Autodesk Inventor part; units mm, degrees
ref_plane "YZ Plane" through (0, 0, 0) normal (1, 0, 0) x (0, 1, 0)
ref_plane "XZ Plane" through (0, 0, 0) normal (0, 1, 0) x (-1, 0, 0)
ref_plane "XY Plane" through (0, 0, 0) normal (0, 0, 1) x (1, 0, 0)
sketch "Sketch1" plane through (0, 0, 0) normal (0, 1, 0) x (-1, 0, 0)
  line L0 (0, 0) -> (0, -42)
  line L1 (0, -42) -> (12, -42)
  line L2 (12, -42) -> (12, 0)
  line L3 (12, 0) -> (0, 0)
  line L4 (0, -21) -> (0, -26)
  line L5 (0, -21) -> (0, -16)
  line L6 (0, -16) -> (0, -19)
  line L7 (0, -16) -> (0, -13)
  line L8 (0, -26) -> (0, -23)
  line L9 (0, -26) -> (0, -29)
  line L10 (0, -29) -> (12, -29)
  line L11 (0, -13) -> (12, -13)
  line L12 (6.4, -16) -> (12, -16)
  line L13 (6.4, -26) -> (12, -26)
  line L14 (12, -16) -> (8, -16)
  circle A0 centre (8, -16) radius 1.6
  circle A1 centre (8, -26) radius 1.6
  line L15 (12, -26) -> (8, -26)
  dimension "d9" = 3.2
  dimension "d10" = 3.2
  dimension "d0" = 42
  dimension "d1" = 12
  dimension "d2" = 5
  dimension "d3" = 5
  dimension "d4" = 3
  dimension "d5" = 3
  dimension "d6" = 3
  dimension "d7" = 3
  dimension "d8" = 4
extrude "Extrusion1" add sketch "Sketch1" along normal blind 15
sketch "Sketch2" plane through (0, 0, 0) normal (0, -1, 0) x (1, 0, 0)
  line L0 (-12, 0) -> (-12, -42)
  line L1 (-12, -42) -> (-12, 0)
  line L2 (-12, -21) -> (-42, -21)
  circle A0 centre (-42, -21) radius 3.5
  arc A1 (-47, -35.1421) -> (-47, -6.8579) centre (-42, -21) ccw
  line L3 (-42, -21) -> (-47, -21)
  line L4 (-47, -21) -> (-47, -35.1421)
  line L5 (-47, -21) -> (-47, -6.8579)
  line L6 (-42, -36) -> (-12, -42)
  line L7 (-42, -6) -> (-12, 0)
  line L8 (-12, -42) -> (0, -42)
  line L9 (0, -42) -> (0, 0)
  line L10 (0, 0) -> (0, -42)
  line L11 (0, 0) -> (-12, 0)
  circle A2 centre (-8, -16) radius 1.6
  circle A3 centre (-8, -16) radius 1.6
  circle A4 centre (-8, -26) radius 1.6
  circle A5 centre (-8, -26) radius 1.6
  line L12 (-12, -42) -> (-12, -36.5)
  line L13 (-12, 0) -> (-12, -5.5)
  line L14 (-17, -6.5) -> (-32.2985, -9.5597)
  line L15 (-32.2985, -32.4403) -> (-17, -35.5)
  circle A6 centre (-42, -21) radius 5
  line L16 (-12, -21) -> (-17, -21)
  line L17 (-17, -16) -> (-17, -6.5)
  line L18 (-17, -26) -> (-17, -35.5)
  line L19 (-42, -16) -> (-33.9223, -16)
  line L20 (-27.8579, -16) -> (-12, -16)
  line L21 (-42, -26) -> (-33.9223, -26)
  line L22 (-27.8579, -26) -> (-12, -26)
  arc A7 (-47, -29.2536) -> (-47, -12.7464) centre (-42, -21) ccw
  line L23 (-12, -21) -> (-12, -31)
  line L24 (-12, -31) -> (-25, -31)
  line L25 (-25, -31) -> (-25, -41)
  line L26 (-25, -41) -> (0, -41)
  line L27 (-12, -21) -> (-12, -11)
  line L28 (-12, -11) -> (-25, -11)
  line L29 (-25, -11) -> (-25, -1)
  line L30 (-25, -1) -> (0, -1)
  line L31 (0, -1) -> (0, -6)
  line L32 (0, -6) -> (-6, -6)
  line L33 (-25, -1) -> (-25, -6)
  line L34 (-25, -6) -> (-19, -6)
  line L35 (-25, -31) -> (-25, -36)
  line L36 (-25, -36) -> (-19, -36)
  circle A8 centre (-19, -36) radius 2.6
  line L37 (0, -41) -> (0, -36)
  line L38 (0, -36) -> (-6, -36)
  circle A9 centre (-6, -36) radius 2.6
  circle A10 centre (-6, -6) radius 2.6
  circle A11 centre (-19, -6) radius 2.6
  line L39 (-27.8579, -16) -> (-12, -16)
  line L40 (-12, -16) -> (-12, -26)
  line L41 (-12, -26) -> (-27.8579, -26)
  point P0 (-47, -12.9223)
  point P1 (-47, -29.0777)
  dimension "d13" = 30
  dimension "d14" = 7
  dimension "d16" = 30
  dimension "d17" = 5
  dimension "d30" = 5.5
  dimension "d31" = 5.5
  dimension "d32" = 10
  dimension "d33" = 5
  dimension "d36" = 19.3
  dimension "d39" = 10
  dimension "d40" = 13
  dimension "d41" = 10
  dimension "d42" = 25
  dimension "d48" = 10
  dimension "d49" = 13
  dimension "d50" = 10
  dimension "d51" = 25
  dimension "d52" = 5
  dimension "d53" = 6
  dimension "d54" = 6
  dimension "d55" = 5
  dimension "d56" = 6
  dimension "d57" = 5.2
  dimension "d58" = 5
  dimension "d59" = 6
  dimension "d60" = 5.2
  dimension "d61" = 5.2
  dimension "d62" = 5.2
extrude "Extrusion2" add sketch "Sketch2" along normal blind 10 contours A9 | A10 | L0 L30 L9 L26 | L0 L28 L17 A11 L34 L29 L7 L30 | L0 L20 L17 L28 | L30 L7 L0 | L0 L11 L9 L30 | L0 L2 A1 L20 | L28 L29 L14 A11 L17 | L17 L20 A1 L14 L29 L28 | L0 L22 A1 L2 | A11 L14 L17 | L17 L14 A11 | L29 L14 A1 L7 | L0 L24 L18 L22 | A1 L2 A7 L5 | L14 L29 L34 A11 | L0 L26 L6 L25 L36 A8 L18 L24 | L18 L24 L25 L15 A1 L22 | A1 L4 A7 L2 | L9 L8 L0 L26 | L18 A8 L15 L25 L24 | A7 L4 A6 L2 | L2 A6 L5 A7 | L0 L6 L26 | A8 L15 L18 | L18 L15 A8 | L15 L25 L6 A1 | A6 L3 A0 L2 | L2 A0 L3 A6 | A8 L36 L25 L15
extrude "Extrusion6" cut sketch "Sketch2" along normal blind 6 contours A7 L4 A6 L2 | L2 A6 L5 A7 | A6 L3 A0 L2 | L2 A0 L3 A6
extrude "Extrusion7" cut sketch "Sketch2" along normal mid plane 40 contours A9 | A10 | L0 L2 A1 L20 | L0 L22 A1 L2 | A11 L14 L17 | L17 L14 A11 | A8 L15 L18 | L18 L15 A8
extrude "Extrusion8" cut sketch "Sketch2" against normal blind 40 contours A9 | A10 | L0 L30 L9 L26 | L0 L28 L17 A11 L34 L29 L7 L30 | L0 L11 L9 L30 | L28 L29 L14 A11 L17 | L7 L29 L30 | L14 L29 L34 A11 | L0 L26 L6 L25 L36 A8 L18 L24 | L9 L8 L0 L26 | L18 A8 L15 L25 L24 | L26 L25 L6 | A8 L36 L25 L15 | A2 | A4
properties part number "servo_clip_holder2_final"
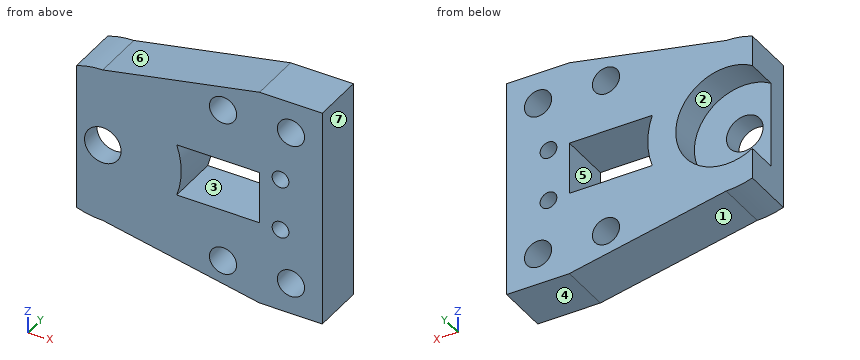
Here's how the part is built. I have some questions about the finished solid (model axes, mm). Face numbers are marked on the shaded views. A direction names the side the tool comes from. Give positions to 0.01 mm unless a question says otherwise; leave off trailing zeros. Loops run counter-clockwise (first coordinate to the right, second up) from the corner with the lowest first, then second, coordinate; pieces in that order, holes last. Notation, with made-up numbers: (48.5, 58) -> (88.5, 58) arc R23 ccw to (88.5, 76) -> close; hole circle Ø4 at (-10.5, 34.25). An arc over 180 degrees is marked (long way). Use one line per item in the form item = value. Start each with the question number.
1) Imagine slicing it at C-C (x = -7.5). Please give me the cut outline in (y, z), then the cut area to 3 significant figures.
2) Thinking about a two-plate mould opening in X: for the marked faces 4, 5, 6 and 7, which applies, +X half, -X half, draft (parallel to the pull), parting line (faces both ways), or undercut?
3) Imagine slicing it at B-B (y = -2.75). Please give me the cut outline in (x, z).
4) Imagine slicing it at A-A (z = -21). Please give me the cut outline in (x, y), then the cut area to 3 significant figures.
5) Please list where these lines run through material, in increasing order: line 1 along Z through (x, y) = (-6, -7); line 2 along X through (y, z) = (-8.4, -21); line 3 along X through (y, z) = (-1.75, -34).
6) Which directions (+Z, -Z, +X, -X, +Y, -Y) give clear straight access to the entire face, cutting with the end or side of a thin tool? Please do the marked faces 1, 2 and 3.
7) For P1, Ø1, axis at y = -2, z = -18.5, coming from the -X side; P2, Ø3, axis at x = -18.5, y = -6, coming from the -Z side; P3, Ø3, axis at x = -16.5, y = -2.5, coming from the +Z side, each with a flat end and sliding along its axis, tell me the tip position at first contact or that it passes through.
8) Imagine slicing it at D-D (y = -9). Count the separate pieces of the cut face and the enclosed holes in it, then the cut area to 3 significant figures.
Check values:
q1.outline = (-10, -42) -> (0, -42) -> (0, -38.12) -> (-10, -38.12) -> close; (-10, -33.88) -> (0, -33.88) -> (0, -27.52) -> (-10, -27.52) -> close; (-10, -24.48) -> (0, -24.48) -> (0, -17.52) -> (-10, -17.52) -> close; (-10, -14.48) -> (0, -14.48) -> (0, -8.12) -> (-10, -8.12) -> close; (-10, -3.88) -> (0, -3.88) -> (0, 0) -> (-10, 0) -> close
q1.area = 274 mm^2
q2.face_4 = draft
q2.face_5 = undercut
q2.face_6 = -X half
q2.face_7 = +X half
q3.outline = (-47, -35.14) arc R15 ccw to (-42, -36) -> (-12, -42) -> (0, -42) -> (0, 0) -> (-12, 0) -> (-42, -6) arc R15 ccw to (-47, -6.86) -> (-47, -12.75) arc R9.65 cw (long way) to (-47, -29.25) -> close; hole (-27.86, -26) -> (-12, -26) -> (-12, -16) -> (-27.86, -16) arc R15 cw to start; hole circle Ø5.2 at (-19, -36); hole circle Ø5.2 at (-19, -6); hole circle Ø3.2 at (-8, -26); hole circle Ø3.2 at (-8, -16); hole circle Ø5.2 at (-6, -36); hole circle Ø5.2 at (-6, -6)
q4.outline = (-47, -10) -> (-45.5, -10) -> (-45.5, -6) -> (-47, -6) -> close; (-38.5, -10) -> (-27, -10) -> (-27, 0) -> (-32.35, 0) -> (-32.35, -6) -> (-38.5, -6) -> close; (-12, -10) -> (0, -10) -> (0, 0) -> (-12, 0) -> close
q4.area = 204 mm^2
q5.line_1 = -42 to -38.6, -33.4 to -8.6, -3.4 to 0
q5.line_2 = -47 to -45.5, -38.5 to -27, -12 to 0
q5.line_3 = -47 to -20.66, -17.34 to -7.66, -4.34 to 0
q6.face_1 = -Z, -X, +Y, -Y
q6.face_2 = +Y
q6.face_3 = +Y, -Y
q7.P1 = -32.83
q7.P2 = -41
q7.P3 = -0.6
q8.separate_pieces = 1
q8.enclosed_holes = 8
q8.area = 1,440 mm^2
